Check sheet for the modelled part. Datum: model origin and axes. Units: mm. Give positions to 0.01 mm unless a question says otherwise; leave off trailing zeros. Order: outer loops, then holes, each group sorted by start corner. A loop starts at its lowest first (then second) coordinate and runs counter-clockwise, first axis right, second up. Notation, with made-up numbers: (81.25, -15) - (109.25, -15) arc R21 ccw to (109.25, 13) - close; hole circle Ø2 at (62, 81). An arc over 180 degrees is marked (long way). Answer in a Markdown table with one row per item.
from build123d import *

# Parameters (mm, degrees)
SKETCH_1_W          = 320
SKETCH_1_H          = 566
SKETCH_1_R          = 2.25
EXTRUDE_1_DEPTH     = 3
SKETCH_3_W          = 191
SKETCH_3_H          = 77
CUT_EXTRUDE_2_DEPTH = 4
SKETCH3_R           = 2.25
CUT_EXTRUDE1_DEPTH  = 4
SKETCH_4_R          = 2.25
SKETCH_4_W          = 28
SKETCH_4_H          = 47
CUT_EXTRUDE_3_DEPTH = 4
FILLET_1_R          = 1.5
SKETCH_5_R          = 4
CUT_EXTRUDE_4_DEPTH = 4
FILLET_2_R          = 1.5


with BuildPart() as part:
    # Эскиз1 → Бобышка-Вытянуть1 (new body)
    with BuildSketch(Plane.XY):
        with Locations((160, 283)):
            Rectangle(SKETCH_1_W, SKETCH_1_H)
        with Locations((10, 553)):
            Circle(SKETCH_1_R, mode=Mode.SUBTRACT)
        with Locations((10, 418)):
            Circle(SKETCH_1_R, mode=Mode.SUBTRACT)
        with Locations((10, 283)):
            Circle(SKETCH_1_R, mode=Mode.SUBTRACT)
        with Locations((10, 148)):
            Circle(SKETCH_1_R, mode=Mode.SUBTRACT)
        with Locations((10, 13)):
            Circle(SKETCH_1_R, mode=Mode.SUBTRACT)
        with Locations((310, 13)):
            Circle(SKETCH_1_R, mode=Mode.SUBTRACT)
        with Locations((160, 553)):
            Circle(SKETCH_1_R, mode=Mode.SUBTRACT)
        with Locations((310, 553)):
            Circle(SKETCH_1_R, mode=Mode.SUBTRACT)
        with Locations((310, 418)):
            Circle(SKETCH_1_R, mode=Mode.SUBTRACT)
        with Locations((310, 283)):
            Circle(SKETCH_1_R, mode=Mode.SUBTRACT)
        with Locations((310, 148)):
            Circle(SKETCH_1_R, mode=Mode.SUBTRACT)
        with Locations((160, 13)):
            Circle(SKETCH_1_R, mode=Mode.SUBTRACT)
    extrude(amount=EXTRUDE_1_DEPTH)

    # Эскиз3 → Вырез-Вытянуть2 (cut, through all)
    with BuildSketch(Plane(origin=(0, 0, 0), x_dir=(-1, 0, 0), z_dir=(0, 0, -1))):
        with Locations((-115.5, 172.5)):
            Rectangle(SKETCH_3_W, SKETCH_3_H)
    extrude(amount=-CUT_EXTRUDE_2_DEPTH, mode=Mode.SUBTRACT)

    # Sketch3 → Cut-Extrude1 (cut, through all)
    with BuildSketch(Plane(origin=(0, 0, 0), x_dir=(-1, 0, 0), z_dir=(0, 0, -1))):
        with Locations((-101, 163)):
            Circle(SKETCH3_R)
        with Locations((-221, 283)):
            Circle(SKETCH3_R)
    extrude(amount=-CUT_EXTRUDE1_DEPTH, mode=Mode.SUBTRACT)

    # Эскиз4 → Вырез-Вытянуть3 (cut, through all)
    with BuildSketch(Plane.XY.offset(3)):
        with Locations((255, 506)):
            Circle(SKETCH_4_R)
        with Locations((295, 506)):
            Circle(SKETCH_4_R)
        with Locations((275, 506)):
            Rectangle(SKETCH_4_W, SKETCH_4_H)
    extrude(amount=-CUT_EXTRUDE_3_DEPTH, mode=Mode.SUBTRACT)

    # Скругление1
    fillet_1_edges = [part.edges().sort_by_distance(p)[0] for p in [
        (211, 211, 1.5),
        (20, 211, 1.5),
        (20, 134, 1.5),
        (211, 134, 1.5),
    ]]
    fillet(fillet_1_edges, radius=FILLET_1_R)

    # Эскиз5 → Вырез-Вытянуть4 (cut, through all)
    with BuildSketch(Plane(origin=(0, 0, 0), x_dir=(-1, 0, 0), z_dir=(0, 0, -1))):
        with Locations((-172.5, 381)):
            Circle(SKETCH_5_R)
        with Locations((-172.5, 358.5)):
            Circle(SKETCH_5_R)
        with Locations((-180.985281374, 372.514718626)):
            Circle(SKETCH_5_R)
        with Locations((-183.75, 361.514428415)):
            Circle(SKETCH_5_R)
        with Locations((-191.985571585, 369.75)):
            Circle(SKETCH_5_R)
        with Locations((-195, 381)):
            Circle(SKETCH_5_R)
        with Locations((-191.985571585, 392.25)):
            Circle(SKETCH_5_R)
        with Locations((-183.75, 400.485571585)):
            Circle(SKETCH_5_R)
        with Locations((-172.5, 403.5)):
            Circle(SKETCH_5_R)
        with Locations((-161.25, 400.485571585)):
            Circle(SKETCH_5_R)
        with Locations((-153.014428415, 392.25)):
            Circle(SKETCH_5_R)
        with Locations((-150, 381)):
            Circle(SKETCH_5_R)
        with Locations((-153.014428415, 369.75)):
            Circle(SKETCH_5_R)
        with Locations((-161.25, 361.514428415)):
            Circle(SKETCH_5_R)
        with Locations((-184.091109915, 384.105828541)):
            Circle(SKETCH_5_R)
        with Locations((-175.605828541, 392.591109915)):
            Circle(SKETCH_5_R)
        with Locations((-164.014718626, 389.485281374)):
            Circle(SKETCH_5_R)
        with Locations((-160.908890085, 377.894171459)):
            Circle(SKETCH_5_R)
        with Locations((-169.394171459, 369.408890085)):
            Circle(SKETCH_5_R)
        with Locations((-68.5, 381)):
            Circle(SKETCH_5_R)
        with Locations((-68.5, 358.5)):
            Circle(SKETCH_5_R)
        with Locations((-76.985281374, 372.514718626)):
            Circle(SKETCH_5_R)
        with Locations((-79.75, 361.514428415)):
            Circle(SKETCH_5_R)
        with Locations((-87.985571585, 369.75)):
            Circle(SKETCH_5_R)
        with Locations((-91, 381)):
            Circle(SKETCH_5_R)
        with Locations((-87.985571585, 392.25)):
            Circle(SKETCH_5_R)
        with Locations((-79.75, 400.485571585)):
            Circle(SKETCH_5_R)
        with Locations((-68.5, 403.5)):
            Circle(SKETCH_5_R)
        with Locations((-57.25, 400.485571585)):
            Circle(SKETCH_5_R)
        with Locations((-49.014428415, 392.25)):
            Circle(SKETCH_5_R)
        with Locations((-46, 381)):
            Circle(SKETCH_5_R)
        with Locations((-49.014428415, 369.75)):
            Circle(SKETCH_5_R)
        with Locations((-57.25, 361.514428415)):
            Circle(SKETCH_5_R)
        with Locations((-80.091109915, 384.105828541)):
            Circle(SKETCH_5_R)
        with Locations((-71.605828541, 392.591109915)):
            Circle(SKETCH_5_R)
        with Locations((-60.014718626, 389.485281374)):
            Circle(SKETCH_5_R)
        with Locations((-56.908890085, 377.894171459)):
            Circle(SKETCH_5_R)
        with Locations((-65.394171459, 369.408890085)):
            Circle(SKETCH_5_R)
    extrude(amount=-CUT_EXTRUDE_4_DEPTH, mode=Mode.SUBTRACT)

    # Скругление2
    fillet_2_edges = [part.edges().sort_by_distance(p)[0] for p in [
        (261, 482.5, 1.5),
        (261, 529.5, 1.5),
        (289, 529.5, 1.5),
        (289, 482.5, 1.5),
    ]]
    fillet(fillet_2_edges, radius=FILLET_2_R)


solid = part.part
(1) Thickness scan on L1, parallel to Y at x = 263, z = 0.5; L2, parallel to Y at x = 195, z = 1.65; L3, parallel to X at y = 386.5, z = 0.9. Record the ranges inside material, lowest first.
Geometry says:
| item | result |
|---|---|
| L1 | 0 to 482.5, 529.5 to 566 |
| L2 | 0 to 134, 211 to 367.12, 372.38 to 377, 385 to 389.62, 394.88 to 566 |
| L3 | 0 to 57.35, 62.68 to 76.89, 83.3 to 161.35, 166.68 to 180.89, 187.3 to 320 |
(2) Cross-section at B-B, the plane x = 32. Record the cut outline in (y, z).
Geometry says:
| item | result |
|---|---|
| outline | (0, 0) - (134, 0) - (134, 3) - (0, 3) - close; (211, 0) - (566, 0) - (566, 3) - (211, 3) - close |
(3) Cross-section at A-A, the plane x = 275.5. Record the cut outline in (y, z), then the cut area to 3 significant figures.
Geometry says:
| item | result |
|---|---|
| outline | (0, 0) - (482.5, 0) - (482.5, 3) - (0, 3) - close; (529.5, 0) - (566, 0) - (566, 3) - (529.5, 3) - close |
| area | 1,560 mm² |
(4) Cross-section at C-C, the plane z = 0.9. Give the number of separate pieces and of enclosed holes in the cut face, then the cut area to 3 significant figures.
Geometry says:
| item | result |
|---|---|
| separate pieces | 1 |
| enclosed holes | 55 |
| area | 163,000 mm² |
